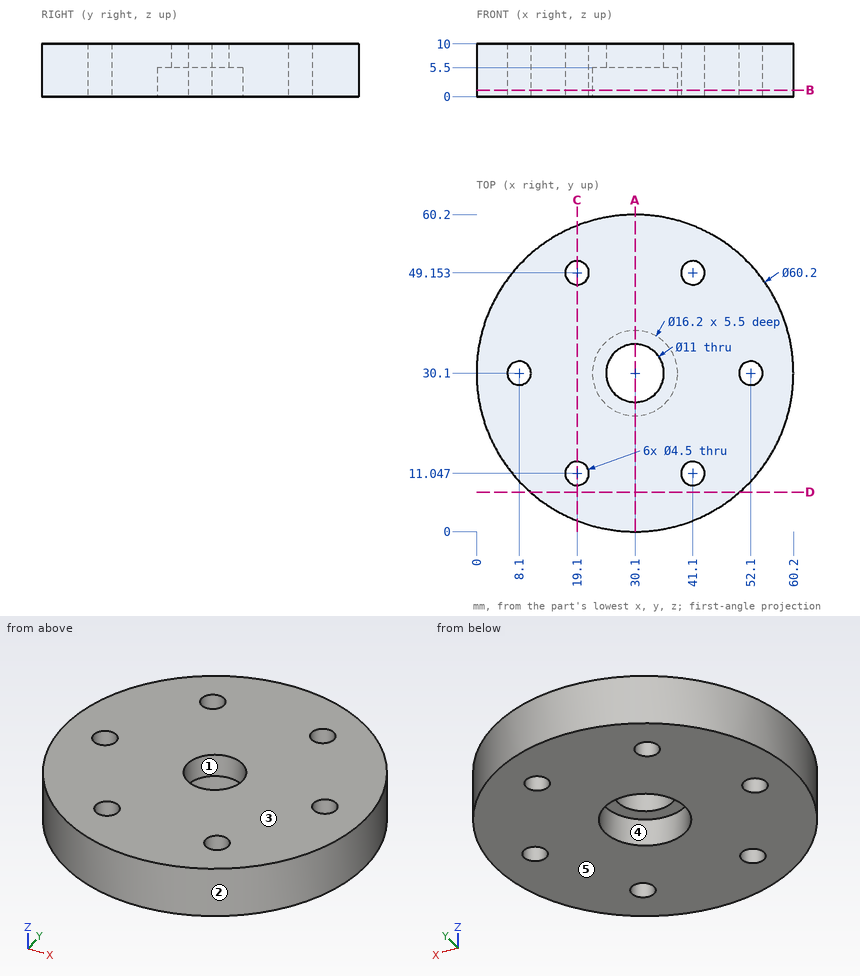
Input: dimensioned drawing with shaded views. Units: mm. Origin: part minimum x, y, z. A direction names the side the tool comes from. Give positions to 0.01 mm unless a question says otherwise; leave off trailing zeros. Loops run counter-clockwise (first coordinate to the right, second up) from the corner with the lowest first, then second, coordinate; pieces in that order, holes last. Notation, with made-up numbers: (74.5, 76) -> (117.5, 76) arc R19 cw to (117.5, 109) -> close; hole circle Ø3 at (86.5, 31). An arc over 180 degrees is marked (long way). Return JSON: item names as keys, results as strings.
Item 1: Section A-A, the plane x = 30.1. Output: boundary loops of the cut face in (y, z).
Filled in:
{"outline": "(0, 0) -> (22, 0) -> (22, 5.5) -> (24.6, 5.5) -> (24.6, 10) -> (0, 10) -> close; (35.6, 5.5) -> (38.2, 5.5) -> (38.2, 0) -> (60.2, 0) -> (60.2, 10) -> (35.6, 10) -> close"}
Item 2: Access query for the marked faces 4 and 5. Directions: +Z, -Z, +X, -X, +Y, -Y. A direction counts if a zero-diameter tool reaches every point of the face in a straight line with its end or side. Return the directions, or none.
Filled in:
{"face 4": "-Z", "face 5": "-Z, +X, -X, +Y, -Y"}
Item 3: Line query: line 1 (X direction, y = 49.5, z = 8.5) (1 decimal); line 2 (Y direction, x = 41.1, z = 5); line 3 (Y direction, x = 30.1, z = 6.7). Output: solid intervals per line, ascending.
Filled in:
{"line 1": "7.1 to 16.9, 21.3 to 38.9, 43.3 to 53.1", "line 2": "2.08 to 8.8, 13.3 to 46.9, 51.4 to 58.12", "line 3": "0 to 24.6, 35.6 to 60.2"}
Item 4: Section C-C, the plane x = 19.1. Output: boundary loops of the cut face in (y, z).
Filled in:
{"outline": "(2.08, 0) -> (8.8, 0) -> (8.8, 10) -> (2.08, 10) -> close; (13.3, 0) -> (46.9, 0) -> (46.9, 10) -> (13.3, 10) -> close; (51.4, 0) -> (58.12, 0) -> (58.12, 10) -> (51.4, 10) -> close"}
Item 5: Pin query (flat end, axial travel): P1, Ø8, axis at x = 27, y = 33.5, coming from the -Z side; P2, Ø2.5, axis at x = 52.1, y = 30.1, coming from the +Z side; P3, Ø5, axis at y = 8.5, z = 8.5, coming from the -X side (1 decimal); P4, Ø5, axis at x = 29, z = 2.5, coming from the -Y side. Return the tip coordinate at first contact, or that it passes through.
Filled in:
{"P1": "z = 0", "P2": "through", "P3": "x = 6.8", "P4": "y = 0"}
Item 6: Section B-B, the plane z = 1.25. Output: boundary loops of the cut face in (x, y).
Filled in:
{"outline": "circle Ø60.2 at (30.1, 30.1); hole circle Ø4.5 at (8.1, 30.1); hole circle Ø4.5 at (19.1, 11.05); hole circle Ø4.5 at (19.1, 49.15); hole circle Ø16.2 at (30.1, 30.1); hole circle Ø4.5 at (41.1, 11.05); hole circle Ø4.5 at (41.1, 49.15); hole circle Ø4.5 at (52.1, 30.1)"}
Item 7: Mould query, pull axis Y, two halves, no side actions, for the marked faces 1, 2 and 3. Classes: released by +Y, released by -Y, zero draft, split by the parting line, or undercut.
Filled in:
{"face 1": "undercut", "face 2": "split by the parting line", "face 3": "zero draft"}
Item 8: Section D-D, the plane y = 7.5. Output: boundary loops of the cut face in (x, z).
Filled in:
{"outline": "(10.22, 0) -> (49.98, 0) -> (49.98, 10) -> (10.22, 10) -> close"}
